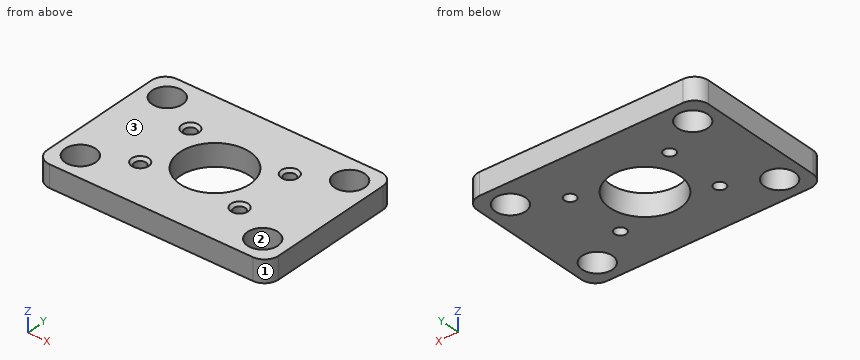
```python
from build123d import *

# Parameters (mm, degrees)
SKETCH1_W           = 41.91
SKETCH1_H           = 27.94
SKETCH1_R           = 2.75
SKETCH1_R_2         = 1.05
SKETCH1_R_3         = 6.35
BOSS_EXTRUDE1_DEPTH = 4
FILLET1_R           = 2.54
CHAMFER1_SIZE       = 0.5


with BuildPart() as part:
    # Sketch1 → Boss-Extrude1 (new body)
    with BuildSketch(Plane.XY):
        Rectangle(SKETCH1_W, SKETCH1_H)
        with Locations((-16.51, 9.525)):
            Circle(SKETCH1_R, mode=Mode.SUBTRACT)
        with Locations((16.51, 9.525)):
            Circle(SKETCH1_R, mode=Mode.SUBTRACT)
        with Locations((16.51, -9.525)):
            Circle(SKETCH1_R, mode=Mode.SUBTRACT)
        with Locations((-16.51, -9.525)):
            Circle(SKETCH1_R, mode=Mode.SUBTRACT)
        with Locations((-9.00049, 5.50037)):
            Circle(SKETCH1_R_2, mode=Mode.SUBTRACT)
        with Locations((9.00049, -5.50037)):
            Circle(SKETCH1_R_2, mode=Mode.SUBTRACT)
        Circle(SKETCH1_R_3, mode=Mode.SUBTRACT)
        with Locations((-9.00049, -5.50037)):
            Circle(SKETCH1_R_2, mode=Mode.SUBTRACT)
        with Locations((9.00049, 5.50037)):
            Circle(SKETCH1_R_2, mode=Mode.SUBTRACT)
    extrude(amount=BOSS_EXTRUDE1_DEPTH)

    # Fillet1
    fillet1_edges = [part.edges().sort_by_distance(p)[0] for p in [
        (-20.955, 13.97, 2),
        (20.955, 13.97, 2),
        (20.955, -13.97, 2),
        (-20.955, -13.97, 2),
    ]]
    fillet(fillet1_edges, radius=FILLET1_R)

    # Chamfer1
    chamfer1_edges = [part.edges().sort_by_distance(p)[0] for p in [
        (7.95049, -5.50037, 4),
        (-10.05049, 5.50037, 4),
        (-10.05049, -5.50037, 4),
        (7.95049, 5.50037, 4),
    ]]
    chamfer(chamfer1_edges, length=CHAMFER1_SIZE)


solid = part.part
```
Read the model definition and answer for the solid it produces. Units are mm, in the model's axes. Face numbers are marked on the shaded views. Give positions to 0.01 mm unless a question says otherwise; leave off trailing zeros. Order: outer loops, then holes, each group sorted by start corner. A loop starts at its lowest first (then second) coordinate and runs counter-clockwise, first axis right, second up. Notation, with made-up numbers: (41, 17) -> (93, 17) arc R26 ccw to (93, 42) -> close; hole circle Ø7 at (17, 9). An arc over 180 degrees is marked (long way). One line per item, written item: value. Start each with the question number.
(1) For a pull along Y with two mould halves and no side action, classify the marked faces 1, 2 and 3 as released by +Y, released by -Y, zero draft, split by the parting line, or undercut.
(2) The part is cut by section A-A (x = -16.51). Determine the outline of the cut face in (y, z) (3 decimals).
(3) The part is cut by section D-D (z = 0.5). State how many separate pieces and enclosed holes the cut face has, and give its area (3 significant figures).
(4) The part is cut by section B-B (x = 0). Determine the outline of the cut face in (y, z), and give its area (3 significant figures).
(5) Straight lines are drawn through the part: L1, parallel to Y at x = 0, z = 3.6; L2, parallel to Y at x = 16.51, z = 2.4 (3 decimals); L3, parallel to X at y = 10.5, z = 2.95 (3 decimals). For each, find the intervals that lie inside material, in ascending order.
(6) A flat-ended cylindrical pin translates along its axis: P1, Ø1.7, axis at x = 9, y = 5.5, coming from the -Z side. Find the tip coordinate at first contact, or state that the pin passes through.
(7) The part is cut by section C-C (y = 0). Determine the outline of the cut face in (x, z) (3 decimals), and give its area (3 significant figures).
Taken from the geometry:
1. face 1: released by -Y
1. face 2: undercut
1. face 3: zero draft
2. outline: (-13.97, 0) -> (-12.275, 0) -> (-12.275, 4) -> (-13.97, 4) -> close; (-6.775, 0) -> (6.775, 0) -> (6.775, 4) -> (-6.775, 4) -> close; (12.275, 0) -> (13.97, 0) -> (13.97, 4) -> (12.275, 4) -> close
3. separate pieces: 1
3. enclosed holes: 9
3. area: 930 mm^2
4. outline: (-13.97, 0) -> (-6.35, 0) -> (-6.35, 4) -> (-13.97, 4) -> close; (6.35, 0) -> (13.97, 0) -> (13.97, 4) -> (6.35, 4) -> close
4. area: 61.0 mm^2
5. L1: -13.97 to -6.35, 6.35 to 13.97
5. L2: -13.97 to -12.275, -6.775 to 6.775, 12.275 to 13.97
5. L3: -20.955 to -19.081, -13.939 to 13.939, 19.081 to 20.955
6. P1: through
7. outline: (-20.955, 0) -> (-6.35, 0) -> (-6.35, 4) -> (-20.955, 4) -> close; (6.35, 0) -> (20.955, 0) -> (20.955, 4) -> (6.35, 4) -> close
7. area: 117 mm^2
